from build123d import *

# Parameters (mm, degrees)
BOSS_EXTRUDE1_REACH                       = 124.544
BOSS_EXTRUDE1_END_RADIUS                  = 37
BOSS_EXTRUDE1_START                       = 25
SKETCH5_R                                 = 19.5
CBORE_START                               = 25
CBORE_FOR_M5_HEX_HEAD_BOLT2_OUTLINE_R     = 11
CBORE_FOR_M5_HEX_HEAD_BOLT2_DEPTH         = 21.000000075
CBORE_START_2                             = 42
CBORE_FOR_M5_HEX_HEAD_BOLT2_2_OUTLINE_R   = 17.5
CBORE_FOR_M5_HEX_HEAD_BOLT2_2_OUTLINE_R_2 = 11
CBORE_FOR_M5_HEX_HEAD_BOLT2_2_DEPTH       = 4.000000075
FILLET1_R                                 = 0.75


# Read off the part's stored shape, not the designer's step: CBORE for M5 Hex Head Bolt2
with BuildPart() as part:
    # Sketch1 → Revolve1 (revolve)
    with BuildSketch(Plane.XY, mode=Mode.PRIVATE) as revolve1_sk:
        with BuildLine():
            Line((0, 72.683334091), (0, 62))
            Line((0, 62), (37, 62))
            Line((37, 62), (37, 0))
            Line((37, 0), (46, 0))
            Line((46, 0), (46, 5))
            Line((46, 5), (42.5, 5))
            Line((42.5, 5), (42.5, 7))
            Line((42.5, 7), (46, 7))
            Line((46, 7), (46, 46))
            Line((46, 46), (42, 46))
            Line((42, 46), (42, 49))
            Line((42, 49), (46, 49))
            Line((46, 49), (46, 51))
            Line((46, 51), (42, 51))
            Line((42, 51), (42, 54))
            Line((42, 54), (46, 54))
            Line((46, 54), (46, 56))
            Line((46, 56), (42, 56))
            Line((42, 56), (42, 59))
            Line((42, 59), (46, 59))
            Line((46, 59), (46, 61))
            Line((46, 61), (42, 61))
            Line((42, 61), (42, 64))
            Line((42, 64), (46, 64))
            Line((46, 64), (46, 67))
            ThreePointArc((46, 67), (23.174880185, 71.257119382), (0, 72.683334091))
        make_face()
    revolve(revolve1_sk.sketch.rotate(Axis((0, 0, 0), (0, 1, 0)), 90), axis=Axis((0, 0, 0), (0, 1, 0)))

    # Boss-Extrude1: up to this cylinder (the profile starts inside it)
    boss_extrude1_end = Plane(origin=(0, 26.5, 0), z_dir=(0, -1, 0)) * Cylinder(BOSS_EXTRUDE1_END_RADIUS, 324.088, mode=Mode.PRIVATE)
    # Sketch5 → Boss-Extrude1 (add, up to the surface)
    with BuildSketch(Plane(origin=(0, 0, 0), x_dir=(0, 0, -1), z_dir=(1, 0, 0)).offset(BOSS_EXTRUDE1_START), mode=Mode.PRIVATE) as boss_extrude1_sk1:
        with Locations(Location((0, 26.5, 0), (0, 0, 180))):
            Circle(SKETCH5_R)
    boss_extrude1_tool1 = extrude(boss_extrude1_sk1.sketch, amount=BOSS_EXTRUDE1_REACH, mode=Mode.PRIVATE) & boss_extrude1_end
    boss_extrude1 = boss_extrude1_tool1.solids().sort_by_distance((25, 26.5, 0))[0]
    add(boss_extrude1)

    # CBORE for M5 Hex Head Bolt2 outline → CBORE for M5 Hex Head Bolt2 (cut)
    with BuildSketch(Plane.YZ.offset(CBORE_START)):
        with Locations((26.5, 0)):
            Circle(CBORE_FOR_M5_HEX_HEAD_BOLT2_OUTLINE_R)
    cbore_for_m5_hex_head_bolt2 = extrude(amount=CBORE_FOR_M5_HEX_HEAD_BOLT2_DEPTH, mode=Mode.SUBTRACT)

    # CBORE for M5 Hex Head Bolt2 2 outline → CBORE for M5 Hex Head Bolt2 2 (cut)
    with BuildSketch(Plane.YZ.offset(CBORE_START_2)):
        with Locations((26.5, 0)):
            Circle(CBORE_FOR_M5_HEX_HEAD_BOLT2_2_OUTLINE_R)
        with Locations((26.5, 0)):
            Circle(CBORE_FOR_M5_HEX_HEAD_BOLT2_2_OUTLINE_R_2, mode=Mode.SUBTRACT)
    cbore_for_m5_hex_head_bolt2_2 = extrude(amount=CBORE_FOR_M5_HEX_HEAD_BOLT2_2_DEPTH, mode=Mode.SUBTRACT)

    # Mirror1: Boss-Extrude1, CBORE for M5 Hex Head Bolt2, CBORE for M5 Hex Head Bolt2 2 across plane
    add(boss_extrude1.mirror(Plane(origin=(0, 0, 0), x_dir=(0, 0, 1), z_dir=(1, 0, 0))))
    add(cbore_for_m5_hex_head_bolt2.mirror(Plane(origin=(0, 0, 0), x_dir=(0, 0, 1), z_dir=(1, 0, 0))), mode=Mode.SUBTRACT)
    add(cbore_for_m5_hex_head_bolt2_2.mirror(Plane(origin=(0, 0, 0), x_dir=(0, 0, 1), z_dir=(1, 0, 0))), mode=Mode.SUBTRACT)

    # Fillet1
    fillet1_edges = [part.edges().sort_by_distance(p)[0] for p in [
        (0, 7, 46),
        (0, 7, 42.5),
        (0, 5, 42.5),
        (0, 5, 46),
    ]]
    fillet(fillet1_edges, radius=FILLET1_R)


solid = part.part
Work out the finished part from the listing and answer in its coordinate system (mm). A direction names the side the tool comes from. Round coordinates to 2 decimals unless told otherwise and drop trailing zeros. Write each loop counter-clockwise with the first axis right and the second up, starting at its lowest first coordinate (ties: lowest second). Pieces come first, ordered by that corner, then holes.
1) Given pin 1 Ø11.5 at (y, z) = (22.5, 1) entering from -X; pin 2 Ø10.5 at (y, z) = (19.5, 1.5) entering from -X; pin 3 Ø2 at (x, z) = (-2, -21) entering from -Y; pin 4 Ø12 at (x, y) = (19.5, 16.5) entering from +Z, each flat-ended and moving along its own axis, determine where each tip first touches the part or whether it passes through.
2) A cutting plane is placed at B-B (z = 0). Give the number of separate pieces and of enclosed holes in the cut face, plus the area to 3 significant figures.
3) A tool of negligible diameter and unlimited length cuts with its end or side. For faces 5 (the cylindrical face through (43.528, 12.613, -10.648)), 6 (the flat face through (-25, 35, 8)), 7 (the flat face through (37.3, 56, -20.2)), from which of +Z, -Z, +X, -X, +Y, -Y can it reach the whole face along a straight path? Write none if from no direction.
4) A cutting plane is placed at A-A (y = 26.5). Give the vertices of the cut face in (x, z).
5) The mould has two halves that part along Z. Classify faces 1 (the flat face through (25, 35, 8)), 2 (the flat face through (37.3, 54, 20.2)), 3 (the cylindrical face through (-12.62, 62.52, -40.06)), 4 (the cylindrical face through (-29.58, 38.37, -15.47)): pulls with the +Z half, pulls with the -Z half, needs draft (parallel to the pull), parting line crosses it, or undercut.
6) A cutting plane is placed at D-D (y = 17). Give the vertices of the cut face in (x, z).
7) Straight lines are drawn through the part: line 1 (Z direction, x = -29, y = 26); line 2 (Y direction, x = -37, z = -22.5); line 3 (X direction, y = 58, z = -19.5). For each, find the intervals that lie inside material, in ascending order.
Completed:
1. pin 1: passes through
1. pin 2: stops at x = -42
1. pin 3: stops at y = 62
1. pin 4: stops at z = 43.97
2. separate pieces: 3
2. enclosed holes: 0
2. area: 1,720 mm2
3. face 5: +X
3. face 6: -Y
3. face 7: none
4. outline: (-42.54, -17.5) arc R46 ccw to (42.54, -17.5) - (42, -17.5) - (42, -11) - (25, -11) - (25, -19.5) - (31.44, -19.5) arc R37 cw to (-31.44, -19.5) - (-25, -19.5) - (-25, -11) - (-42, -11) - (-42, -17.5) - close; (-42.54, 17.5) - (-42, 17.5) - (-42, 11) - (-25, 11) - (-25, 19.5) - (-31.44, 19.5) arc R37 cw to (31.44, 19.5) - (25, 19.5) - (25, 11) - (42, 11) - (42, 17.5) - (42.54, 17.5) arc R46 ccw to start
5. face 1: undercut
5. face 2: needs draft
5. face 3: parting line crosses it
5. face 4: undercut
6. outline: (-43.59, -14.7) arc R46 ccw to (43.59, -14.7) - (42, -14.7) - (42, -5.55) - (25, -5.55) - (25, -17.03) - (32.85, -17.03) arc R37 cw to (-32.85, -17.03) - (-25, -17.03) - (-25, -5.55) - (-42, -5.55) - (-42, -14.7) - close; (-43.59, 14.7) - (-42, 14.7) - (-42, 5.55) - (-25, 5.55) - (-25, 17.03) - (-32.85, 17.03) arc R37 cw to (32.85, 17.03) - (25, 17.03) - (25, 5.55) - (42, 5.55) - (42, 14.7) - (43.59, 14.7) arc R46 ccw to start
7. line 1: z = -35.71 to -22.98, -19.49 to -10.99, 10.99 to 19.49, 22.98 to 35.71
7. line 2: y = 0 to 5, 7 to 46, 49 to 51, 54 to 56, 59 to 61, 64 to 67.66
7. line 3: x = -37.2 to -31.44, 31.44 to 37.2
